Autodesk Inventor part; units mm, degrees
ref_plane "YZ Plane" through (0, 0, 0) normal (1, 0, 0) x (0, 1, 0)
ref_plane "XZ Plane" through (0, 0, 0) normal (0, 1, 0) x (-1, 0, 0)
ref_plane "XY Plane" through (0, 0, 0) normal (0, 0, 1) x (1, 0, 0)
sketch "Sketch1" plane through (0, 0, 0) normal (1, 0, 0) x (0, 1, 0)
  line L0 (0, 0) -> (100, 0)
  line L1 (100, 0) -> (100, -350)
  line L2 (100, -350) -> (0, -350)
  line L3 (0, -350) -> (0, 0)
  dimension "d0" = 100
  dimension "d1" = 350
extrude "Extrusion1" add sketch "Sketch1" along normal blind 0.607
sketch "Sketch2" plane through (0.607, 0, 0) normal (1, 0, 0) x (0, 0, -1)
  line L0 (350, 100) -> (0, 100)
  line L1 (0, 100) -> (175, 100)
  line L2 (175, 100) -> (175, 75)
  circle A0 centre (175, 75) radius 7.5
  line L3 (175, 75) -> (87.5, 75)
  line L4 (175, 75) -> (262.5, 75)
  circle A1 centre (87.5, 75) radius 7.5
  circle A2 centre (262.5, 75) radius 7.5
  point P0 (0, 0)
  dimension "d4" = 175
  dimension "d5" = 25
  dimension "d6" = 15
  dimension "d10" = 15
  dimension "d11" = 15
  dimension "d12" = 87.5
extrude "Extrusion2" cut sketch "Sketch2" against normal through all
equation "\"BendRadius\" = Thickness"
equation "\"BendReliefWidth\" = Thickness"
equation "\"BendReliefDepth\" = 0.5 * Thickness"
equation "\"CornerReliefSize\" = 4 * Thickness"
equation "\"MinimumRemnant\" = 2 * Thickness"
equation "\"TransitionRadius\" = BendRadius"
equation "\"JacobiRadiusSize\" = BendRadius"
equation "\"GapSize\" = Thickness"
properties part number "project support plate small" material "Steel, Galvanized"
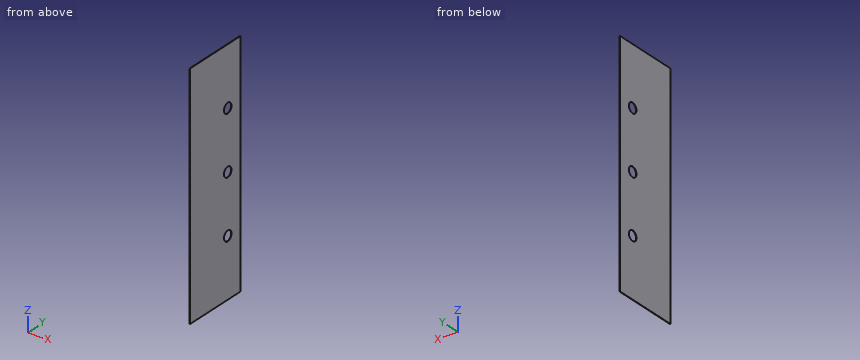
Check sheet for the modelled part. Datum: model origin and axes. Units: mm. Round coordinates to 2 decimals unless told otherwise and drop trailing zeros. Order: outer loops, then holes, each group sorted by start corner. A loop starts at its lowest first (then second) coordinate and runs counter-clockwise, first axis right, second up. Notation, with made-up numbers: (26.5, -23.5) -> (47.5, -23.5) arc R23 ccw to (47.5, -1.5) -> close; hole circle Ø8 at (2, -14.5). An arc over 180 degrees is marked (long way). One line per item, written item: value. Start each with the question number.
Q1. Thickness scan on line 1 (Y direction, x = 0.2, z = -175); line 2 (Y direction, x = 0.45, z = -168.5). Record the ranges inside material, lowest first.
Q2. Cross-section at C-C (x = 0.15). Record the boundary of the cut face in (y, z).
Q3. Cross-section at D-D (z = -87). Record the boundary of the cut face in (x, y).
Q4. Cross-section at A-A (y = 75). Record the boundary of the cut face in (x, z), and give its area (3 significant figures).
Q5. Cross-section at B-B (z = -262.5). Record the boundary of the cut face in (x, y).
Q6. Gauge pin test, flat end, axial feed: pin 1 Ø13.5 at (y, z) = (75, -175) entering from +X. Record the tip position at first contact, or that the pin passes through.
Completed:
1. line 1: y = 0 to 67.5, 82.5 to 100
1. line 2: y = 0 to 71.26, 78.74 to 100
2. outline: (0, -350) -> (100, -350) -> (100, 0) -> (0, 0) -> close; hole circle Ø15 at (75, -262.5); hole circle Ø15 at (75, -175); hole circle Ø15 at (75, -87.5)
3. outline: (0, 0) -> (0.61, 0) -> (0.61, 67.52) -> (0, 67.52) -> close; (0, 82.48) -> (0.61, 82.48) -> (0.61, 100) -> (0, 100) -> close
4. outline: (0, -350) -> (0.61, -350) -> (0.61, -270) -> (0, -270) -> close; (0, -255) -> (0.61, -255) -> (0.61, -182.5) -> (0, -182.5) -> close; (0, -167.5) -> (0.61, -167.5) -> (0.61, -95) -> (0, -95) -> close; (0, -80) -> (0.61, -80) -> (0.61, 0) -> (0, 0) -> close
4. area: 185 mm²
5. outline: (0, 0) -> (0.61, 0) -> (0.61, 67.5) -> (0, 67.5) -> close; (0, 82.5) -> (0.61, 82.5) -> (0.61, 100) -> (0, 100) -> close
6. pin 1: passes through
